Input: part model. Units: mm. Frame: model coordinates. Face numbers are marked on the shaded views. A direction names the side the tool comes from. Coordinates: 2 decimals unless noted, no trailing zeros. Loops run counter-clockwise (first coordinate to the right, second up) from the corner with the lowest first, then second, coordinate; pieces in that order, holes last. Notation, with made-up numbers: (29, -11.5) -> (47, -11.5) arc R24 cw to (47, 16.5) -> close; hole circle Ø2 at (71.25, 79.5). An arc over 180 degrees is marked (long way). Put each result on its own line as item: value. Start each with the question number.
1) Cut plane A-A (y = 0). Return the cut outline in (x, z), plus the area to 3 significant figures.
2) Cut plane D-D (z = 7.75). State how many separate pieces and enclosed holes the cut face has, plus the area to 3 significant figures.
3) Pull-direction query (X, two-part tool) for the marked faces 1, 2 and 3; classes: pulls with the +X half, pulls with the -X half, needs draft (parallel to the pull), parting line crosses it, or undercut.
4) Material intervals for L1, parallel to Y at x = 18.5, z = 5; L2, parallel to Y at x = 7, z = 7.5; L3, parallel to X at y = 0, z = 3.55, sorted ascending.
5) Cut plane C-C (x = 8.5). Return the cut outline in (y, z).
6) Contact query for flat-ended pins moving along their axis: P1, Ø0.8, axis at x = 18, y = 7, coming from the +Z side; P2, Ø12, axis at x = 6.5, y = 1, coming from the +Z side; P3, Ø2.5, axis at x = 20.5, z = 4.5, coming from the +Y side. Output: stop coordinate, or through.
7) Set-up query: the marked faces 4, 5, 6, 7 and 8. Return all of +Z, -Z, +X, -X, +Y, -Y with unobstructed straight access to the full face (end or side cutting, diameter ignored); none if empty.
from build123d import *
from build123d.topology import SkipClean

# Parameters (mm, degrees)
SKETCH1_R                        = 1.75
BOSS_EXTRUDE1_DEPTH              = 7.5
SKETCH2_R                        = 1.75
BOSS_EXTRUDE2_DEPTH              = 2.5
SKETCH3_W                        = 1.5
SKETCH3_H                        = 2
CUT_EXTRUDE1_DEPTH               = 4.5
SKETCH4_R                        = 3
CUT_EXTRUDE2_DEPTH               = 3.5
M1_6_CLEARANCE_HOLE1_OUTLINE_R   = 0.9
M1_6_CLEARANCE_HOLE1_DEPTH       = 9
M1_6_START                       = 6
M1_6_CLEARANCE_HOLE1_2_OUTLINE_R = 0.9
M1_6_CLEARANCE_HOLE1_2_DEPTH     = 3


# Read off the part's stored shape, not the designer's step: M1.6 Clearance Hole1
with BuildPart() as part:
    # Sketch1 → Boss-Extrude1 (new body)
    with BuildSketch(Plane.XY.offset(1.5)):
        with BuildLine():
            Line((18.85, -9.5), (-18.85, -9.5))
            Line((-18.85, -9.5), (-18.85, -8))
            Line((-18.85, -8), (-13.35, -8))
            Line((-13.35, -8), (-13.35, -7))
            Line((-13.35, -7), (-10.35, -7))
            Line((-10.35, -7), (-10.35, -8))
            Line((-10.35, -8), (17.35, -8))
            Line((17.35, -8), (17.35, 9))
            Line((17.35, 9), (-10.35, 9))
            Line((-10.35, 9), (-10.35, 7))
            Line((-10.35, 7), (-13.35, 7))
            Line((-13.35, 7), (-13.35, 8))
            Line((-13.35, 8), (-13.84, 8))
            Line((-13.84, 8), (-18.85, 8))
            Line((-18.85, 8), (-18.85, 9.5))
            Line((-18.85, 9.5), (-13.84, 9.5))
            ThreePointArc((-13.84, 9.5), (-13.493517677, 9.643517677), (-13.35, 9.99))
            Line((-13.35, 9.99), (-13.35, 10.01))
            ThreePointArc((-13.35, 10.01), (-13.206482323, 10.356482323), (-12.86, 10.5))
            Line((-12.86, 10.5), (18.85, 10.5))
            Line((18.85, 10.5), (18.85, 9.5))
            Line((18.85, 9.5), (18.85, 5))
            Line((18.85, 5), (23.6, 5))
            ThreePointArc((23.6, 5), (28.35, 0), (23.6, -5))
            Line((23.6, -5), (18.85, -5))
            Line((18.85, -5), (18.85, -9.5))
        make_face()
        with Locations((23.343421053, 0)):
            Circle(SKETCH1_R, mode=Mode.SUBTRACT)
    extrude(amount=BOSS_EXTRUDE1_DEPTH)

    # Sketch2 → Boss-Extrude2 (add)
    with SkipClean():  # the faces are left unmerged after this step: merging them gives an invalid solid
        with BuildSketch(Plane.XY):
            with BuildLine():
                Line((-18.85, 8), (-18.85, -8))
                Line((-18.85, -8), (-18.85, -9.5))
                Line((-18.85, -9.5), (18.85, -9.5))
                Line((18.85, -9.5), (18.85, -5))
                Line((18.85, -5), (23.6, -5))
                ThreePointArc((23.6, -5), (28.35, 0), (23.6, 5))
                Line((23.6, 5), (18.85, 5))
                Line((18.85, 5), (18.85, 10.5))
                Line((18.85, 10.5), (-12.86, 10.5))
                ThreePointArc((-12.86, 10.5), (-13.206482323, 10.356482323), (-13.35, 10.01))
                Line((-13.35, 10.01), (-13.35, 9.99))
                ThreePointArc((-13.35, 9.99), (-13.493517677, 9.643517677), (-13.84, 9.5))
                Line((-13.84, 9.5), (-18.85, 9.5))
                Line((-18.85, 9.5), (-18.85, 8))
            make_face()
            with Locations((23.343421053, 0)):
                Circle(SKETCH2_R, mode=Mode.SUBTRACT)
        extrude(amount=BOSS_EXTRUDE2_DEPTH)
    add(part.part.scale(1), mode=Mode.REPLACE)  # the faces are merged on a copy

    # Sketch3 → Cut-Extrude1 (cut)
    with BuildSketch(Plane.XY.offset(9)):
        with Locations((18.1, 7)):
            Rectangle(SKETCH3_W, SKETCH3_H)
    extrude(amount=-CUT_EXTRUDE1_DEPTH, mode=Mode.SUBTRACT)

    # Sketch4 → Cut-Extrude2 (cut)
    with BuildSketch(Plane.XY.offset(9)):
        with Locations((23.343421053, 0)):
            Circle(SKETCH4_R)
    extrude(amount=-CUT_EXTRUDE2_DEPTH, mode=Mode.SUBTRACT)

    # M1.6 Clearance Hole1 outline → M1.6 Clearance Hole1 (cut)
    with BuildSketch(Plane.XY):
        with Locations((17.15, 8.8)):
            Circle(M1_6_CLEARANCE_HOLE1_OUTLINE_R)
        with Locations((17.15, -7.8)):
            Circle(M1_6_CLEARANCE_HOLE1_OUTLINE_R)
    extrude(amount=M1_6_CLEARANCE_HOLE1_DEPTH, mode=Mode.SUBTRACT)

    # M1.6 Clearance Hole1 2 outline → M1.6 Clearance Hole1 2 (cut)
    with BuildSketch(Plane.XY.offset(M1_6_START)):
        with BuildLine():
            Line((-11.437689437, -7), (-12.262310563, -7))
            ThreePointArc((-12.262310563, -7), (-11.85, -8.7), (-11.437689437, -7))
        make_face()
        with Locations((-11.85, 8.8)):
            Circle(M1_6_CLEARANCE_HOLE1_2_OUTLINE_R)
    extrude(amount=M1_6_CLEARANCE_HOLE1_2_DEPTH, mode=Mode.SUBTRACT)


solid = part.part
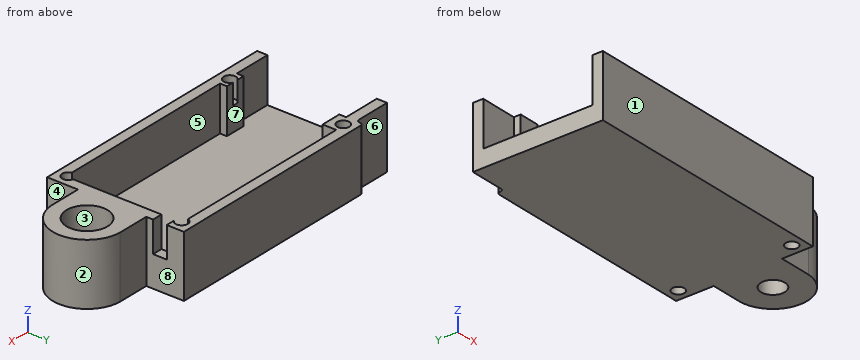
Results found:
1. outline: (-18.85, 0) -> (21.59, 0) -> (21.59, 5.5) -> (20.34, 5.5) -> (20.34, 9) -> (17.35, 9) -> (17.35, 2.5) -> (-18.85, 2.5) -> close; (25.09, 0) -> (28.35, 0) -> (28.35, 9) -> (26.34, 9) -> (26.34, 5.5) -> (25.09, 5.5) -> close
1. area: 149 mm2
2. separate pieces: 2
2. enclosed holes: 2
2. area: 193 mm2
3. face 1: needs draft
3. face 2: pulls with the +X half
3. face 3: undercut
4. L1: y = -9.5 to 6, 8 to 10.5
4. L2: y = -9.5 to -8, 9 to 10.5
4. L3: x = 17.35 to 21.59, 25.09 to 28.35
5. outline: (-9.5, 0) -> (10.5, 0) -> (10.5, 9) -> (9, 9) -> (9, 2.5) -> (-8, 2.5) -> (-8, 9) -> (-9.5, 9) -> close
6. P1: stops at z = 4.5
6. P2: stops at z = 2.5
6. P3: stops at y = 5
7. face 4: +Z, -Z, +X, -Y
7. face 5: +Z
7. face 6: +Z, -Z, -X, +Y
7. face 7: +Z, -X
7. face 8: +Z, -Z, +X, +Y
